from build123d import *

# Parameters (mm, degrees)
SKETCH1_R           = 2.7
BOSS_EXTRUDE1_DEPTH = 2.38125


with BuildPart() as part:
    # Sketch1 → Boss-Extrude1 (new, symmetric)
    with BuildSketch(Plane.XY):
        Polygon((0, 0), (0, 60), (20, 60), (60, 20), (60, 0), align=None)
        with Locations(Location((10, 10, 0), (0, 0, 180))):
            Circle(SKETCH1_R, mode=Mode.SUBTRACT)
        with Locations(Location((49.624, 10, 0), (0, 0, 180))):
            Circle(SKETCH1_R, mode=Mode.SUBTRACT)
        with Locations(Location((10, 49.624, 0), (0, 0, 180))):
            Circle(SKETCH1_R, mode=Mode.SUBTRACT)
    extrude(amount=BOSS_EXTRUDE1_DEPTH, both=True)


solid = part.part
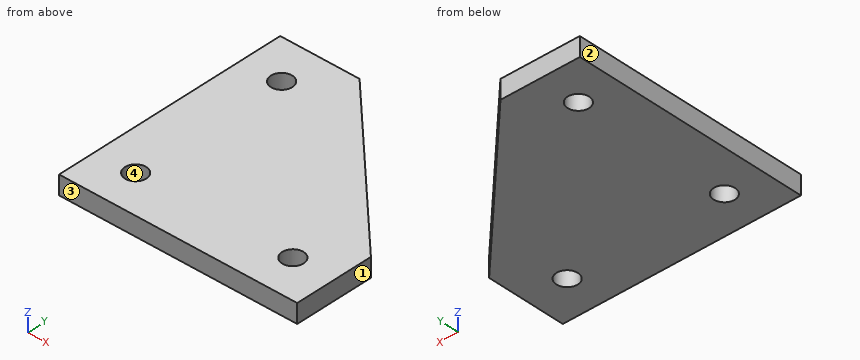
Input: part model. Units: mm. Frame: model coordinates. Face numbers are marked on the shaded views. Give positions to 0.01 mm unless a question says otherwise; leave off trailing zeros. Loops run counter-clockwise (first coordinate to the right, second up) from the corner with the lowest first, then second, coordinate; pieces in that order, holes last. Notation, with made-up numbers: (-11, 1) -> (45, 1) arc R17 cw to (45, 13) -> close; hole circle Ø9 at (42, 67). An arc over 180 degrees is marked (long way). Answer as a JSON object with one key per item and string values. Group by question number.
Item 1: Cut plane C-C, the plane z = 1.35. Return the cut outline in (x, y).
Item 2: Pull-direction query (X, two-part tool) for the marked faces 1, 2, 3 and 4; classes: released by +X, released by -X, zero draft, split by the parting line, or undercut.
Item 3: Line query: probe 1 along Y at (x, z) = (10, 0.85); probe 2 along Y at (x, z) = (56, 1.95). Output: solid intervals per line, ascending.
Item 4: Cut plane D-D, the plane x = 28.5. Return the cut outline in (y, z), and give its area (3 significant figures).
Item 5: Cut plane A-A, the plane x = 10. Return the cut outline in (y, z).
Checks:
{
 "1": {"outline": "(0, 0) -> (60, 0) -> (60, 20) -> (20, 60) -> (0, 60) -> close; hole circle Ø5.4 at (10, 10); hole circle Ø5.4 at (10, 49.62); hole circle Ø5.4 at (49.62, 10)"},
 "2": {"face 1": "released by +X", "face 2": "released by -X", "face 3": "zero draft", "face 4": "undercut"},
 "3": {"probe 1": "y = 0 to 7.3, 12.7 to 46.92, 52.32 to 60", "probe 2": "y = 0 to 24"},
 "4": {"outline": "(0, -2.38) -> (51.5, -2.38) -> (51.5, 2.38) -> (0, 2.38) -> close", "area": "245 mm²"},
 "5": {"outline": "(0, -2.38) -> (7.3, -2.38) -> (7.3, 2.38) -> (0, 2.38) -> close; (12.7, -2.38) -> (46.92, -2.38) -> (46.92, 2.38) -> (12.7, 2.38) -> close; (52.32, -2.38) -> (60, -2.38) -> (60, 2.38) -> (52.32, 2.38) -> close"}
}
